Can you work these out from the model? Positions are in its coordinate system, mm. Give positions to 0.01 mm unless a question says otherwise; leave off trailing zeros. Write each loop counter-clockwise with the first axis right and the second up, starting at its lowest first coordinate (ties: lowest second). Pieces come first, ordered by that corner, then holes.
1. If I drill on probe 1 along X at (y, z) = (14, -50.5); probe 2 along Z at (x, y) = (-8.5, 7); probe 3 along X at (y, z) = (25, -53), over which ranges is the centre line in solid material (lowest first)?
2. Suppose I cut it at B-B (y = 4.5). Please give me the cut outline in (x, z).
3. Suppose I cut it at A-A (y = 15). Please give me the cut outline in (x, z).
4. Suppose I cut it at C-C (x = -6). Give the number of separate pieces and of enclosed holes in the cut face, and give its area (3 significant figures).
5. Thinking about a two-plate mould opening in X: for faces 1 (the cylindrical face through (19.61, 15.21, -41.08)), 2 (the cylindrical face through (-35.75, 15.18, -63.98)), 3 (the cylindrical face through (18.49, 29.4, -33.17)), which applies, pulls with the +X half, pulls with the -X half, needs draft (parallel to the pull), parting line crosses it, or undercut?
6. I'm going to push flat-ended pins straight in: pin 1 (1 mm diameter, centred on x = -4.5, z = -10.5, fed in from +Y); pin 2 (4 mm diameter, centred on x = -7.5, y = 21, fed in from +Z); pin 3 (6 mm diameter, centred on y = 3.5, z = -40, fed in from -X); pin 4 (12 mm diameter, centred on x = -15, z = -49.95, fed in from -Y). Where does each tip first touch, or does it pass through?
```python
from build123d import *

# Parameters (mm, degrees)
BOSS_EXTRUDE1_DEPTH = 30
FILLET1_R           = 2
SKETCH2_R           = 10
CUT_EXTRUDE3_DEPTH  = 31
SKETCH3_R           = 5
CUT_EXTRUDE4_DEPTH  = 73.07179677


with BuildPart() as part:
    # Sketch1 → Boss-Extrude1 (new body)
    with BuildSketch(Plane(origin=(0, 0, 0), x_dir=(1, 0, 0), z_dir=(0, 1, 0))):
        Polygon((0, 0), (37.5, 64.951905284), (-37.5, 64.951905284), align=None)
    extrude(amount=BOSS_EXTRUDE1_DEPTH)

    # Fillet1
    fillet1_edges = [part.edges().sort_by_distance(p)[0] for p in [
        (0, 30, -64.951905284),
        (0, 0, -64.951905284),
        (-18.75, 30, -32.475952642),
        (18.75, 0, -32.475952642),
        (-18.75, 0, -32.475952642),
        (-37.5, 15, -64.951905284),
        (37.5, 15, -64.951905284),
        (0, 15, 0),
        (18.75, 30, -32.475952642),
    ]]
    fillet(fillet1_edges, radius=FILLET1_R)

    # Sketch2 → Cut-Extrude3 (cut, through all)
    with BuildSketch(Plane(origin=(0, 30, 0), x_dir=(1, 0, 0), z_dir=(0, 1, 0))):
        with Locations((-15, 49.951905284)):
            Circle(SKETCH2_R)
        with Locations((15, 49.951905284)):
            Circle(SKETCH2_R)
        with Locations((0, 33.951905284)):
            Circle(SKETCH2_R)
    extrude(amount=-CUT_EXTRUDE3_DEPTH, mode=Mode.SUBTRACT)

    # Sketch3 → Cut-Extrude4 (cut, through all)
    with BuildSketch(Plane.ZY.offset(36.035898385)):
        with Locations((-33.951905284, 15)):
            Circle(SKETCH3_R)
    extrude(amount=-CUT_EXTRUDE4_DEPTH, mode=Mode.SUBTRACT)


solid = part.part
```
Checks:
1. probe 1: x = -29.16 to -24.98, -5.02 to 5.02, 24.98 to 29.16
1. probe 2: z = -64.95 to -57.55, -42.35 to -39.22, -28.68 to -14.72
1. probe 3: x = -30.6 to -24.52, -5.48 to 5.48, 24.52 to 30.6
2. outline: (-35.77, -61.95) arc R2 ccw to (-34.04, -64.95) - (34.04, -64.95) arc R2 ccw to (35.77, -61.95) - (1.73, -3) arc R2 ccw to (-1.73, -3) - close; hole circle Ø20 at (-15, -49.95); hole circle Ø20 at (0, -33.95); hole circle Ø20 at (15, -49.95)
3. outline: (-35.77, -61.95) arc R2 ccw to (-34.04, -64.95) - (34.04, -64.95) arc R2 ccw to (35.77, -61.95) - (22.49, -38.95) - (8.66, -38.95) arc R10 cw to (-8.66, -38.95) - (-22.49, -38.95) - close; (-16.72, -28.95) - (-8.66, -28.95) arc R10 cw to (8.66, -28.95) - (16.72, -28.95) - (1.73, -3) arc R2 ccw to (-1.73, -3) - close; hole circle Ø20 at (-15, -49.95); hole circle Ø20 at (15, -49.95)
4. separate pieces: 3
4. enclosed holes: 0
4. area: 890 mm2
5. face 1: undercut
5. face 2: pulls with the -X half
5. face 3: pulls with the +X half
6. pin 1: stops at y = 29.99
6. pin 2: stops at z = -9.53
6. pin 3: stops at x = -24.83
6. pin 4: passes through
